from build123d import *

# Parameters (mm, degrees)
EXTRUDE_THIN1_DEPTH     = 228.6
CUT_EXTRUDE1_DEPTH      = 1
CUT_EXTRUDE1_DEPTH_BACK = 39.1


with BuildPart() as part:
    # Sketch1 → Extrude-Thin1 (new body, symmetric)
    with BuildSketch(Plane.XY):
        with BuildLine():
            Line((-15.875, 19.05), (15.875, 19.05))
            ThreePointArc((15.875, 19.05), (18.12006403, 18.12006403), (19.05, 15.875))
            Line((19.05, 15.875), (19.05, -15.875))
            ThreePointArc((19.05, -15.875), (18.12006403, -18.12006403), (15.875, -19.05))
            Line((15.875, -19.05), (-15.875, -19.05))
            ThreePointArc((-15.875, -19.05), (-18.12006403, -18.12006403), (-19.05, -15.875))
            Line((-19.05, -15.875), (-19.05, 15.875))
            ThreePointArc((-19.05, 15.875), (-18.12006403, 18.12006403), (-15.875, 19.05))
        make_face()
        with BuildLine():
            Line((-15.875, 16.51), (15.875, 16.51))
            ThreePointArc((15.875, 16.51), (16.324012806, 16.324012806), (16.51, 15.875))
            Line((16.51, 15.875), (16.51, -15.875))
            ThreePointArc((16.51, -15.875), (16.324012806, -16.324012806), (15.875, -16.51))
            Line((15.875, -16.51), (-15.875, -16.51))
            ThreePointArc((-15.875, -16.51), (-16.324012806, -16.324012806), (-16.51, -15.875))
            Line((-16.51, -15.875), (-16.51, 15.875))
            ThreePointArc((-16.51, 15.875), (-16.324012806, 16.324012806), (-15.875, 16.51))
        make_face(mode=Mode.SUBTRACT)
    extrude(amount=EXTRUDE_THIN1_DEPTH, both=True)

    # Sketch3 → Cut-Extrude1 (cut, two sides)
    with BuildSketch(Plane(origin=(0, 19.05, 0), x_dir=(1, 0, 0), z_dir=(0, 1, 0))) as cut_extrude1_sk:
        Polygon((890.680220904, -545.847455696), (19.05, -228.6), (-19.05, -214.732734074), (-890.680220904, 102.514721621), (-1525.175132295, -1640.745720186), (256.185309512, -2289.107897503), align=None)
    extrude(amount=CUT_EXTRUDE1_DEPTH, mode=Mode.SUBTRACT)
    extrude(cut_extrude1_sk.sketch, amount=-CUT_EXTRUDE1_DEPTH_BACK, mode=Mode.SUBTRACT)


solid = part.part
Design review of the part built by this model. Coordinates are the model's own, in mm. A direction names the side the tool comes from. Give positions to 0.01 mm unless a question says otherwise; leave off trailing zeros. Loops run counter-clockwise (first coordinate to the right, second up) from the corner with the lowest first, then second, coordinate; pieces in that order, holes last. Notation, with made-up numbers: (-35.75, 59.5) - (-13.75, 59.5) arc R12 cw to (-13.75, 74.5) - close; hole circle Ø7 at (-1, -6). An arc over 180 degrees is marked (long way). Write item = value, one per line.
1) Take a section at B-B on z = 112. State the section outline as (x, y) points (3 decimals), and give its area (3 significant figures).
Result sheet:
outline = (-19.05, -15.875) arc R3.175 ccw to (-15.875, -19.05) - (15.875, -19.05) arc R3.175 ccw to (19.05, -15.875) - (19.05, 15.875) arc R3.175 ccw to (15.875, 19.05) - (-15.875, 19.05) arc R3.175 ccw to (-19.05, 15.875) - close; hole (-16.51, -15.875) arc R0.635 ccw to (-15.875, -16.51) - (15.875, -16.51) arc R0.635 ccw to (16.51, -15.875) - (16.51, 15.875) arc R0.635 ccw to (15.875, 16.51) - (-15.875, 16.51) arc R0.635 ccw to (-16.51, 15.875) - close
area = 353 mm2
2) To check wall thickness, follow line 1 (Y direction, x = -13, z = 122). State the ranges of the line that lie inside material, in increasing order.
Result sheet:
line_1 = -19.05 to -16.51, 16.51 to 19.05
3) Take a section at A-A on y = 10. State the section outline as (x, z) points.
Result sheet:
outline = (-19.05, -228.6) - (-16.51, -228.6) - (-16.51, 215.66) - (-19.05, 214.73) - close; (16.51, -228.6) - (19.05, -228.6) - (19.05, 228.6) - (16.51, 227.68) - close
4) Take a section at C-C on x = 9. State the section outline as (y, z) points.
Result sheet:
outline = (-19.05, -228.6) - (-16.51, -228.6) - (-16.51, 224.94) - (-19.05, 224.94) - close; (16.51, -228.6) - (19.05, -228.6) - (19.05, 224.94) - (16.51, 224.94) - close
5) Draft analysis for pull direction X (two halves, no side actions). For faces 1 (the face through (-16.51, 0, -3)), 2 (the face through (0.267, -16.667, 221.763)), 3 (the face through (0, 19.05, 3)), state which applies: +X half, -X half, draft (parallel to the pull), parting line (faces both ways), or undercut.
Result sheet:
face_1 = undercut
face_2 = -X half
face_3 = draft
6) Tool access review of faces 4 (the face through (16.51, 0, 3)), 5 (the face through (19.05, 0, 3)): name each direction out of +Z, -Z, +X, -X, +Y, -Y from which nothing blocks a thin tool from reaching the whole face with its end or side.
Result sheet:
face_4 = +Z, -Z
face_5 = +Z, -Z, +X, +Y, -Y
